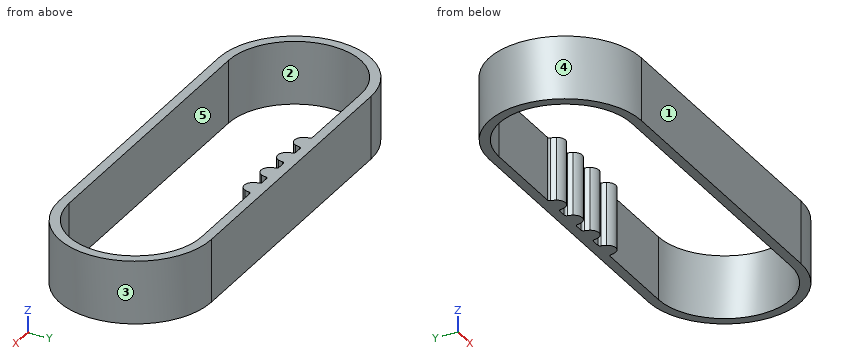
```python
from build123d import *

# Parameters (mm, degrees)
BOSS_EXTRUDE1_DEPTH = 2
BOSS_EXTRUDE2_DEPTH = 2
LPATTERN1_COUNT     = 2
LPATTERN1_PITCH     = 4


with BuildPart() as part:
    # Sketch1 → Boss-Extrude1 (new body, symmetric)
    with BuildSketch(Plane.XY):
        with BuildLine():
            Line((0, 4.831), (19.004204728, 4.831))
            ThreePointArc((19.004204728, 4.831), (23.835204728, 0), (19.004204728, -4.831))
            Line((19.004204728, -4.831), (0, -4.831))
            ThreePointArc((0, -4.831), (-4.831, 0), (0, 4.831))
        make_face()
        with BuildLine():
            Line((0, 4.201), (19.004204728, 4.201))
            ThreePointArc((19.004204728, 4.201), (23.205204728, 0), (19.004204728, -4.201))
            Line((19.004204728, -4.201), (0, -4.201))
            ThreePointArc((0, -4.201), (-4.201, 0), (0, 4.201))
        make_face(mode=Mode.SUBTRACT)
    extrude(amount=BOSS_EXTRUDE1_DEPTH, both=True)

    # Sketch2 → Boss-Extrude2 (add, symmetric)
    with BuildSketch(Plane.XY):
        with BuildLine():
            Line((5.502102364, 4.831), (5.502102364, 4.201))
            Line((5.502102364, 4.201), (5.761926939, 4.201))
            ThreePointArc((5.761926939, 4.201), (5.86083401, 4.163771412), (5.910645473, 4.070565217))
            ThreePointArc((5.910645473, 4.070565217), (5.94449065, 3.912937846), (6.00322596, 3.762797753))
            ThreePointArc((6.00322596, 3.762797753), (6.502102364, 3.451), (7.000978769, 3.762797753))
            ThreePointArc((7.000978769, 3.762797753), (7.059714078, 3.912937846), (7.093559256, 4.070565217))
            ThreePointArc((7.093559256, 4.070565217), (7.143370718, 4.163771412), (7.242277789, 4.201))
            Line((7.242277789, 4.201), (7.761926939, 4.201))
            ThreePointArc((7.761926939, 4.201), (7.86083401, 4.163771412), (7.910645473, 4.070565217))
            ThreePointArc((7.910645473, 4.070565217), (7.94449065, 3.912937846), (8.00322596, 3.762797753))
            ThreePointArc((8.00322596, 3.762797753), (8.502102364, 3.451), (9.000978769, 3.762797753))
            ThreePointArc((9.000978769, 3.762797753), (9.059714078, 3.912937846), (9.093559256, 4.070565217))
            ThreePointArc((9.093559256, 4.070565217), (9.143370718, 4.163771412), (9.242277789, 4.201))
            Line((9.242277789, 4.201), (9.502102364, 4.201))
            Line((9.502102364, 4.201), (9.502102364, 4.831))
            Line((9.502102364, 4.831), (5.502102364, 4.831))
        make_face()
    boss_extrude2 = extrude(amount=BOSS_EXTRUDE2_DEPTH, both=True)

    # LPattern1: Boss-Extrude2 ×2
    with Locations(*[(i * LPATTERN1_PITCH, 0, 0) for i in range(1, LPATTERN1_COUNT)]):
        add(boss_extrude2)


solid = part.part
```
Work out the finished part from the listing and answer in its coordinate system (mm). Face numbers are marked on the shaded views. A direction names the side the tool comes from. Round coordinates to 2 decimals unless told otherwise and drop trailing zeros. Order: outer loops, then holes, each group sorted by start corner. A loop starts at its lowest first (then second) coordinate and runs counter-clockwise, first axis right, second up.
Q1. A cutting plane is placed at B-B, the plane x = 1.75. Determine the outline of the cut face in (y, z).
Solution:
outline: (-4.83, -2) - (-4.2, -2) - (-4.2, 2) - (-4.83, 2) - close; (4.2, -2) - (4.83, -2) - (4.83, 2) - (4.2, 2) - close
Q2. A tool of negligible diameter and unlimited length cuts with its end or side. For the marked faces 4 and 5, from which of +Z, -Z, +X, -X, +Y, -Y can it reach the whole face along a straight path? Write none if from no direction.
Solution:
face 4: +Z, -Z, -X
face 5: +Z, -Z
Q3. The mould has two halves that part along X. Classify the marked faces 1, 2 and 3: pulls with the +X half, pulls with the -X half, needs draft (parallel to the pull), parting line crosses it, or undercut.
Solution:
face 1: needs draft
face 2: undercut
face 3: pulls with the +X half
Q4. A cutting plane is placed at A-A, the plane y = 0. Determine the outline of the cut face in (x, z), then the cut area to 3 significant figures.
Solution:
outline: (-4.83, -2) - (-4.2, -2) - (-4.2, 2) - (-4.83, 2) - close; (23.21, -2) - (23.84, -2) - (23.84, 2) - (23.21, 2) - close
area: 5.04 mm2
Q5. Find the intervals of material crossed by line 1 along Y through (x, z) = (15.5, -0.35); line 2 along Y through (x, z) = (6, 0.25); line 3 along X through (y, z) = (-3.25, -0.45), in increasing order.
Solution:
line 1: y = -4.83 to -4.2, 4.2 to 4.83
line 2: y = -4.83 to -4.2, 3.77 to 4.83
line 3: x = -3.57 to -2.66, 21.67 to 22.58
